The figure shows three views and two pictorial views of one solid part (mm, origin at its lowest corner). Answer the questions. A direction names the side the tool comes from. Coordinates: 2 decimals unless noted, no trailing zeros. Loops run counter-clockwise (first coordinate to the right, second up) from the corner with the lowest first, then second, coordinate; pieces in that order, holes last. Notation, with made-up numbers: M -9.5,62.5 L 8.5,62.5 A20 cw 8.5,74.5 Z; hole C 21,29 d6. An arc over 180 degrees is marked long. Answer as a JSON object with one key per item and string values. Group by question number.
1. A cutting plane is placed at A-A on x = 15.82. Give the vertices of the cut face in (y, z) (3 decimals).
2. For the marked faces 1 and 2, determine the directions among +Z, -Z, +X, -X, +Y, -Y from which every point of the face is accessible in a straight line to the end or side of a thin tool.
3. A cutting plane is placed at D-D on z = 11. Give the vertices of the cut face in (x, y) (3 decimals).
4. Determine the mould class of the marked faces 3, 4 and 5 for opening direction X: released by +X, released by -X, zero draft, split by the parting line, or undercut.
5. Straight lines are drawn through the part: L1, parallel to Z at x = 8, y = 5; L2, parallel to Z at x = 15.82, y = 26.95; L3, parallel to X at y = 15, z = 11.25. For each, find the intervals that lie inside material, in ascending order.
6. Given pin 1 (5 mm diameter, centred on x = 15.82, z = 14.2, fed in from -Y) (3 decimals); pin 2 (4 mm diameter, centred on x = 5.5, z = 4.5, fed in from -Y); pin 3 (3 mm diameter, centred on y = 24.5, z = 10.5, fed in from +X); pin 4 (13 mm diameter, centred on x = 15.82, y = 15.82, fed in from +Z), each flat-ended and moving along its own axis, determine where each tip first touches the part or whether it passes through.
7. A cutting plane is placed at B-B on y = 15.82. Give the vertices of the cut face in (x, z) (3 decimals), and give its area (3 significant figures).
8. A cutting plane is placed at C-C on z = 15.25. Give the vertices of the cut face in (x, y) (3 decimals).
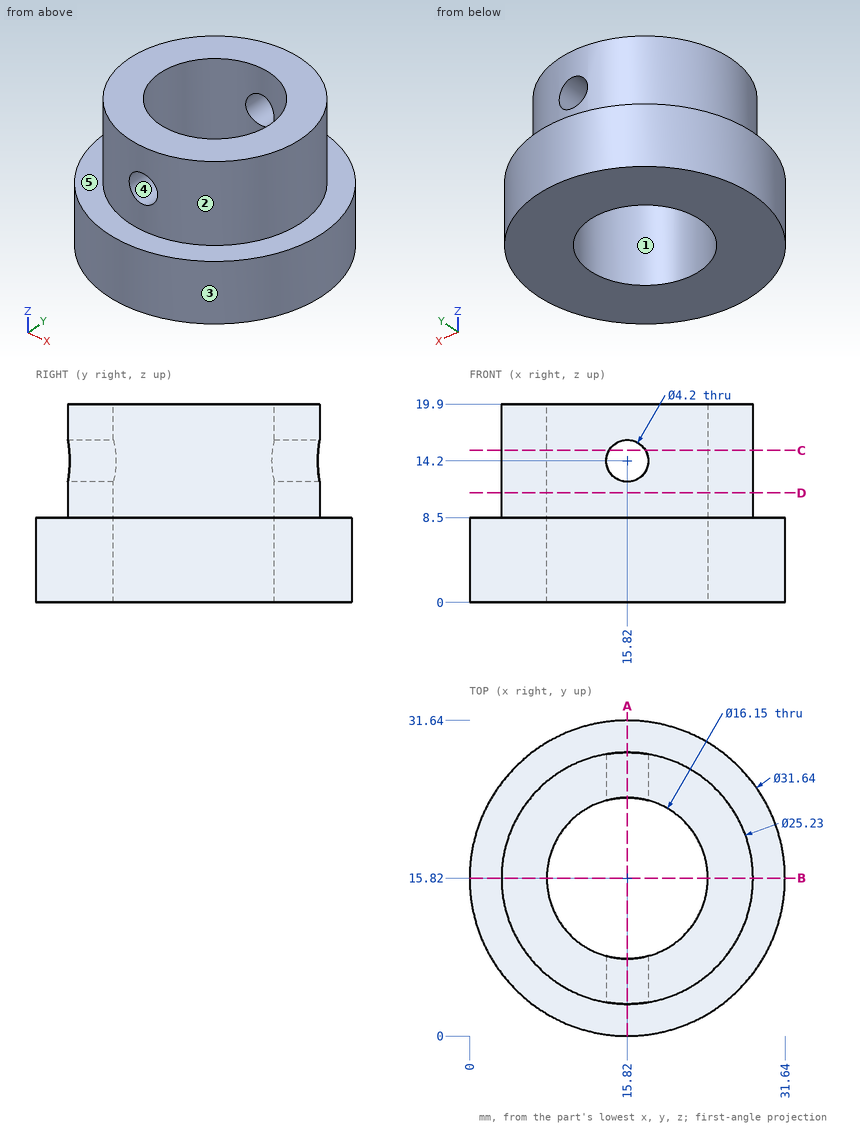
From the geometry:
{
 "1": {"outline": "M 0,0 L 7.745,0 L 7.745,12.1 L 3.205,12.1 L 3.205,8.5 L 0,8.5 Z; M 3.205,16.3 L 7.745,16.3 L 7.745,19.9 L 3.205,19.9 Z; M 23.895,0 L 31.64,0 L 31.64,8.5 L 28.435,8.5 L 28.435,12.1 L 23.895,12.1 Z; M 23.895,16.3 L 28.435,16.3 L 28.435,19.9 L 23.895,19.9 Z"},
 "2": {"face 1": "+Z, -Z", "face 2": "+Z"},
 "3": {"outline": "C 15.82,15.82 d25.23; hole C 15.82,15.82 d16.15"},
 "4": {"face 3": "split by the parting line", "face 4": "undercut", "face 5": "zero draft"},
 "5": {"L1": "z = 0 to 8.5", "L2": "z = 0 to 12.1, 16.3 to 19.9", "L3": "x = 3.23 to 7.79, 23.85 to 28.41"},
 "6": {"pin 1": "stops at y = 3.205", "pin 2": "stops at y = 2.36", "pin 3": "stops at x = 26.19", "pin 4": "passes through"},
 "7": {"outline": "M 0,0 L 7.745,0 L 7.745,19.9 L 3.205,19.9 L 3.205,8.5 L 0,8.5 Z; M 23.895,0 L 31.64,0 L 31.64,8.5 L 28.435,8.5 L 28.435,19.9 L 23.895,19.9 Z", "area": "235 mm²"},
 "8": {"outline": "M 14.001,3.337 L 14.001,7.952 A8.075 cw 14.001,23.688 L 14.001,28.303 A12.615 ccw Z; M 17.639,3.337 A12.615 ccw 17.639,28.303 L 17.639,23.688 A8.075 cw 17.639,7.952 Z"}
}
